Geometry check sheet. Reference: drawing and pictorial views, mm from the part's lowest x, y, z. Round coordinates to 2 decimals unless told otherwise and drop trailing zeros. Write each loop counter-clockwise with the first axis right and the second up, starting at its lowest first coordinate (ties: lowest second). Pieces come first, ordered by that corner, then holes. Notation, with made-up numbers: M 69.25,38.5 L 117.25,38.5 A27 ccw 117.25,70.5 Z; hole C -23.5,46 d6. An arc over 180 degrees is marked long. Put each result on its own line as item: value. Start each with the question number.
(1) Section check B-B on z = 44. Count the separate pieces of the cut face and the enclosed holes in it.
(2) Material ranges on probe 1 along X at (y, z) = (1.15, 47); probe 2 along X at (y, z) = (1.1, 6.5); probe 3 along X at (y, z) = (0.7, 9.5), recorded low to high.
(3) Section check A-A on y = 1.25. Record the cut outline in (x, z).
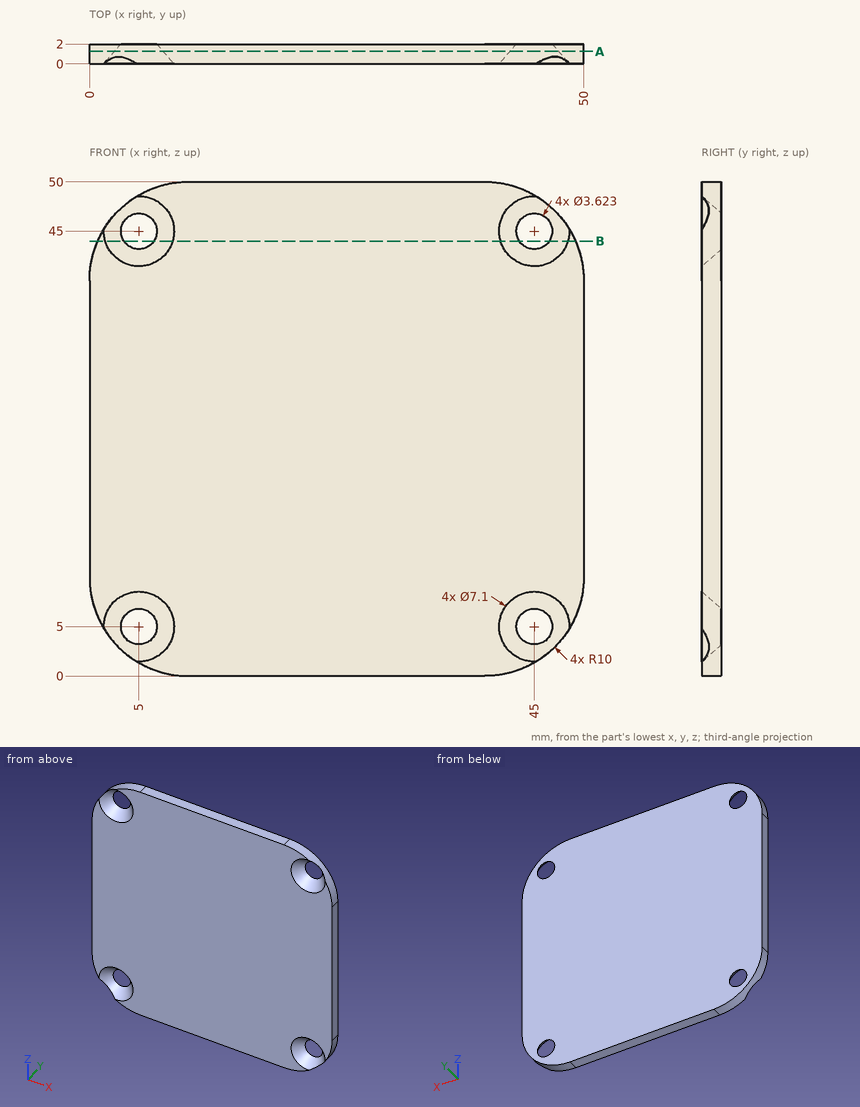
Answers follow:
1. separate pieces: 3
1. enclosed holes: 0
2. probe 1: x = 2.86 to 3.42, 6.58 to 43.42, 46.58 to 47.14
2. probe 2: x = 0.63 to 2.88, 7.12 to 42.88, 47.12 to 49.37
2. probe 3: x = 0.01 to 49.99
3. outline: M 0,10 A10 ccw 10,0 L 40,0 A10 ccw 50,10 L 50,40 A10 ccw 40,50 L 10,50 A10 ccw 0,40 Z; hole C 5,5 d4.93; hole C 5,45 d4.93; hole C 45,5 d4.93; hole C 45,45 d4.93
